For this review, take the finished solid that the model builds, in its own axes (mm). Give positions to 0.01 mm unless a question says otherwise; leave off trailing zeros. Write each loop counter-clockwise with the first axis right and the second up, starting at its lowest first coordinate (ties: lowest second). Pieces come first, ordered by that corner, then holes. Notation, with made-up numbers: (0, 48.5) -> (24, 48.5) arc R16 ccw to (24, 74.5) -> close; hole circle Ø9 at (-16, 34.5). An arc over 180 degrees is marked (long way). Write item = value, one per line.
```python
from build123d import *

# Parameters (mm, degrees)
F1_DEPTH = 30.48
F2_R     = 5.08


with BuildPart() as f1:
    # F0 (on Top) → F1 (new body)
    with BuildSketch(Plane.XY):
        with BuildLine():
            Line((-45.563514, -33.3848), (-41.111397, -45.278859))
            Line((-41.111397, -45.278859), (-36.357604, -57.978859))
            add(Edge.make_bspline(
                [(-36.357604, -57.978859), (-24.389937, -53.096968), (-0.454603, -43.333187), (23.480731, -53.096968), (35.448398, -57.978859)],
                knots=[0, 0, 0, 0, 37.206947, 74.413894, 74.413894, 74.413894, 74.413894], degree=3))
            Line((35.448398, -57.978859), (40.202191, -45.278859))
            Line((40.202191, -45.278859), (44.654308, -33.3848))
            add(Edge.make_bspline(
                [(-45.563514, -33.3848), (-30.527211, -28.382681), (-0.454603, -17.247475), (29.618004, -28.382681), (44.654308, -33.3848)],
                knots=[0, 0, 0, 0, 46.330691, 92.661381, 92.661381, 92.661381, 92.661381], degree=3))
        make_face()
    extrude(amount=F1_DEPTH)

    # F2
    f2_edges = [f1.edges().sort_by_distance(p)[0] for p in [
        (-0.454603, -48.215078, 30.48),
        (-0.454603, -22.815078, 30.48),
    ]]
    fillet(f2_edges, radius=F2_R)


solid = f1.part
```
(1) For pin 1 (1.5 mm diameter, centred on y = -51.5, z = 17, fed in from +X); pin 2 (5 mm diameter, centred on y = -37, z = 17.5, fed in from +X); pin 3 (8 mm diameter, centred on x = 0, z = 16, fed in from -Y), all flat-tipped, find the tip position at first contact; note any pin that passes through.
Answers below:
pin_1 = 38.15
pin_2 = 44.24
pin_3 = -48.43
(2) Take a section at A-A (y = -41). Write out the cut boundary in (x, z).
Answers below:
outline = (-42.71, 0) -> (41.8, 0) -> (41.8, 30.48) -> (-42.71, 30.48) -> close
(3) To check wall thickness, follow probe 1 along Z at (x, y) = (25.5, -52.5); probe 2 along Y at (x, z) = (0, 13.5); probe 3 along Y at (x, z) = (16, 7.5). State the ranges of each line that lie inside material, in increasing order.
Answers below:
probe_1 = 0 to 28.93
probe_2 = -48.22 to -22.82
probe_3 = -50.82 to -24.74
